from build123d import *

# Parameters (mm, degrees)
SKETCH1_R                       = 1.6
BOSS_EXTRUDE1_DEPTH             = 8.8
SKETCH2_W                       = 6.5
SKETCH2_H                       = 10
BOSS_EXTRUDE2_DEPTH             = 3.7
BOSS_EXTRUDE2_DIRECTION_2_REACH = 30.332
SKETCH3_W                       = 6.5
SKETCH3_H                       = 44.6
BOSS_EXTRUDE3_DEPTH             = 4
CHAMFER1_SIZE                   = 2
CHAMFER2_SIZE                   = 1.55


with BuildPart() as part:
    # Sketch1 → Boss-Extrude1 (new body)
    with BuildSketch(Plane.XY):
        Polygon((0, 0), (8, 0), (9.5, 0), (9.5, 25.2), (8, 25.2), (0, 25.2), align=None)
        with Locations((6, 20)):
            Circle(SKETCH1_R, mode=Mode.SUBTRACT)
        with Locations(Location((6, 5.2, 0), (0, 0, 180))):
            Circle(SKETCH1_R, mode=Mode.SUBTRACT)
    extrude(amount=BOSS_EXTRUDE1_DEPTH)

    # Sketch2 → Boss-Extrude2 (add)
    with BuildSketch(Plane.XY.offset(8.8)):
        with Locations((12.75, 5)):
            Rectangle(SKETCH2_W, SKETCH2_H)
    extrude(amount=BOSS_EXTRUDE2_DEPTH)

    # Boss-Extrude2 direction 2: up to this face of the body (flat: up to its plane)
    boss_extrude2_direction_2_end = Plane(part.part.faces().sort_by_distance((4.659964898, 12.6, 0))[0])
    # Sketch2 → Boss-Extrude2 direction 2 (add, up to the picked face)
    with BuildSketch(Plane.XY.offset(8.8), mode=Mode.PRIVATE) as boss_extrude2_direction_2_sk1:
        with Locations((12.75, 5)):
            Rectangle(SKETCH2_W, SKETCH2_H)
    boss_extrude2_direction_2_tool1 = split(extrude(boss_extrude2_direction_2_sk1.sketch, amount=-BOSS_EXTRUDE2_DIRECTION_2_REACH, mode=Mode.PRIVATE), bisect_by=boss_extrude2_direction_2_end, keep=Keep.BOTH, mode=Mode.PRIVATE)
    add(boss_extrude2_direction_2_tool1.solids().sort_by(Axis((12.75, 5, 8.8), (0, 0, -1)))[0])

    # Sketch3 → Boss-Extrude3 (add)
    with BuildSketch(Plane.XY.offset(12.5)):
        with Locations((12.75, 22.3)):
            Rectangle(SKETCH3_W, SKETCH3_H)
    extrude(amount=BOSS_EXTRUDE3_DEPTH)

    # Chamfer1
    chamfer1_edges = [part.edges().sort_by_distance(p)[0] for p in [
        (4.75, 25.2, 8.8),
        (9.5, 0, 12.65),
        (16, 0, 8.25),
        (16, 10, 6.25),
        (9.5, 10, 4.4),
        (9.5, 22.3, 16.5),
        (12.75, 0, 16.5),
        (16, 22.3, 16.5),
        (0, 12.6, 8.8),
        (4.75, 0, 8.8),
    ]]
    chamfer(chamfer1_edges, length=CHAMFER1_SIZE)

    # Chamfer2
    chamfer2_edges = [part.edges().sort_by_distance(p)[0] for p in [
        (4.4, 20, 8.8),
        (7.6, 5.2, 8.8),
    ]]
    chamfer(chamfer2_edges, length=CHAMFER2_SIZE)


solid = part.part
Verification items for the finished model (mm, model axes). A direction names the side the tool comes from. Round coordinates to 2 decimals unless told otherwise and drop trailing zeros. Loops run counter-clockwise (first coordinate to the right, second up) from the corner with the lowest first, then second, coordinate; pieces in that order, holes last. Notation, with made-up numbers: M 0.5,-9 L 32.5,-9 A32 ccw 32.5,23 Z; hole C 51,16.5 d10. An arc over 180 degrees is marked long. Write each question's results on one line, items separated by ' | '.
1) Section check D-D on z = 10.25. Record the boundary of the cut face in (x, y).
Checks:
outline: M 9.5,2 L 11.5,0 L 14,0 L 16,2 L 16,8 L 14,10 L 9.5,10 Z
2) Scan lines: L1, parallel to Y at x = 6, z = 3; L2, parallel to X at y = 5.2, z = 2.25; L3, parallel to Y at x = 6.5, z = 6.75. Record each from-to range of solid material in increasing order. Write a range as from..to.
Checks:
L1: y = 0..3.6, 6.8..18.4, 21.6..25.2 | L2: x = 0..4.4, 7.6..16 | L3: y = 0..3.68, 6.72..18.48, 21.52..25.2
3) Access from +Z, -Z, +X, -X, +Y, -Y to the whole of each face (thin tool, end or side, straight path). Record for faces 5 (the flat face through (5.7, 1, 7.8)), 6 (the flat face through (6, 10, 0)), 7 (the flat face through (9.5, 18, 13)), 8 (the flat face through (12, 10, 8)).
Checks:
face 5: +Z, -X, -Y | face 6: -Z, +X, -X, +Y, -Y | face 7: +Z, -X, +Y, -Y | face 8: +X, +Y
4) Section check C-C on y = 20. Record the boundary of the cut face in (x, z), then the cut area to 3 significant figures.
Checks:
outline: M 0,0 L 4.4,0 L 4.4,7.25 L 2.85,8.8 L 2,8.8 L 0,6.8 Z; M 7.6,0 L 9.5,0 L 9.5,8.8 L 9.15,8.8 L 7.6,7.25 Z; M 9.5,12.5 L 16,12.5 L 16,14.5 L 14,16.5 L 11.5,16.5 L 9.5,14.5 Z | area: 73.0 mm2
5) Gauge pin test, flat ends, axial feed: P1, Ø2, axis at x = 2.5, z = 4.5, coming from the +Y side; P2, Ø5, axis at x = 13, y = 23.5, coming from the -Z side; P3, Ø2, axis at x = 11, z = 9, coming from the +Y side. Record the tip position at first contact, or that the pin passes through.
Checks:
P1: stops at y = 25.2 | P2: stops at z = 12.5 | P3: stops at y = 11.48
6) Section check A-A on y = 5.2. Record the boundary of the cut face in (x, z), then the cut area to 3 significant figures.
Checks:
outline: M 0,0 L 4.4,0 L 4.4,7.25 L 2.85,8.8 L 2,8.8 L 0,6.8 Z; M 7.6,0 L 16,0 L 16,14.5 L 14,16.5 L 11.5,16.5 L 9.5,14.5 L 9.5,8.8 L 9.15,8.8 L 7.6,7.25 Z | area: 154 mm2
7) Mould release check, pull along Y, two halves, no side actions. Record for faces 1 (the flat face through (9.5, 19, 4)), 2 (the flat face through (12.7, 1, 15.5)), 3 (the cylindrical face through (5.792, 21.586, 3.574)), 4 (the flat face through (13, 44.6, 14)): released by +Y, released by -Y, zero draft, split by the parting line, or undercut.
Checks:
face 1: zero draft | face 2: released by -Y | face 3: undercut | face 4: released by +Y
8) Section check B-B on x = 6. Record the boundary of the cut face in (y, z).
Checks:
outline: M 0,0 L 3.6,0 L 3.6,7.25 L 2.05,8.8 L 2,8.8 L 0,6.8 Z; M 6.8,0 L 18.4,0 L 18.4,7.25 L 16.85,8.8 L 8.35,8.8 L 6.8,7.25 Z; M 21.6,0 L 25.2,0 L 25.2,6.8 L 23.2,8.8 L 23.15,8.8 L 21.6,7.25 Z
